Build history of the part. All positions in model axes, mm. A direction names the side the tool comes from. Round coordinates to 2 decimals unless told otherwise and drop trailing zeros. Loops run counter-clockwise (first coordinate to the right, second up) from the corner with the lowest first, then second, coordinate; pieces in that order, holes last. Notation, with made-up numbers: M 84.25,-4.5 L 114.25,-4.5 A26 cw 114.25,18.5 Z; hole C 12.5,65.5 d9. An arc over 180 degrees is marked long. Use one line per item in the form item = value. Start each with the question number.
```python
from build123d import *

# Parameters (mm, degrees)
SKETCH_R        = 1.7
PAD_DEPTH       = 10
SKETCH002_W     = 15
SKETCH002_H     = 10
POCKET_DEPTH    = 7
PAD001_DEPTH    = 3
SKETCH009_R     = 2.8
POCKET003_DEPTH = 2.5
SKETCH010_R     = 1.5
PAD002_DEPTH    = 3
SKETCH011_R     = 1
POCKET004_DEPTH = 24
SKETCH012_R     = 1.8
POCKET005_DEPTH = 11
SKETCH013_R     = 2
POCKET006_DEPTH = 6
FILLET_R        = 2
FILLET001_R     = 2


with BuildPart() as part:
    # Sketch → Pad (new body)
    with BuildSketch(Plane.XY):
        Polygon((-10, 10), (5, 10), (5, 4.942513), (5, -5.057487), (5, -10), (-10, -10), (-10, -5.057487), (-25, -5.057487), (-25, 4.942513), (-10, 4.942513), align=None)
        with Locations((-17.661669, 0)):
            Circle(SKETCH_R, mode=Mode.SUBTRACT)
        with Locations((-7.661669, 0)):
            Circle(SKETCH_R, mode=Mode.SUBTRACT)
    extrude(amount=PAD_DEPTH)

    # Sketch002 (on Face14 of Pad) → Pocket (cut)
    with BuildSketch(Plane.XY.offset(10)):
        with Locations((-17.5, -0.057487)):
            Rectangle(SKETCH002_W, SKETCH002_H)
    extrude(amount=-POCKET_DEPTH, mode=Mode.SUBTRACT)

    # Sketch003 (on Face13 of Pocket) → Pad001 (join)
    with BuildSketch(Plane.XZ.offset(10)):
        with BuildLine():
            ThreePointArc((1.21175, 5.90888), (0, 9.5), (-1.21175, 5.90888))
            Line((-1.21175, 5.90888), (-1.21175, 0))
            Line((-1.21175, 0), (1.21175, 0))
            Line((1.21175, 0), (1.21175, 5.90888))
        make_face()
    extrude(amount=PAD001_DEPTH)

    # Sketch009 (on Face14 of Pad) → Pocket003 (cut)
    with BuildSketch(Plane.XY.offset(10)):
        with Locations((-7.661669, 0)):
            Circle(SKETCH009_R)
    extrude(amount=-POCKET003_DEPTH, mode=Mode.SUBTRACT)

    # Sketch010 (on Face24 of Pocket003) → Pad002 (join)
    with BuildSketch(Plane.XZ.offset(13)):
        with Locations((0, 7.5)):
            Circle(SKETCH010_R)
    extrude(amount=PAD002_DEPTH)

    # Sketch011 (on Face26 of Pad002) → Pocket004 (cut)
    with BuildSketch(Plane.XZ.offset(16)):
        with Locations((0, 7.5)):
            Circle(SKETCH011_R)
    extrude(amount=-POCKET004_DEPTH, mode=Mode.SUBTRACT)

    # Sketch012 (on Face1 of Pocket004) → Pocket005 (cut)
    with BuildSketch(Plane(origin=(-10, 0, 0), x_dir=(0, -1, 0), z_dir=(-1, 0, 0))):
        with Locations((-7.264964, 7)):
            Circle(SKETCH012_R)
    extrude(amount=-POCKET005_DEPTH, mode=Mode.SUBTRACT)

    # Sketch013 (on Face1 of Pocket005) → Pocket006 (cut)
    with BuildSketch(Plane(origin=(-10, 0, 0), x_dir=(0, -1, 0), z_dir=(-1, 0, 0))):
        with Locations((-7.264964, 7)):
            Circle(SKETCH013_R)
    extrude(amount=-POCKET006_DEPTH, mode=Mode.SUBTRACT)

    # Fillet
    fillet_edges = [part.edges().sort_by_distance(p)[0] for p in [
        (5, -10, 5),
    ]]
    fillet(fillet_edges, radius=FILLET_R)

    # Fillet001
    fillet001_edges = [part.edges().sort_by_distance(p)[0] for p in [
        (-25, -0.057487, 3),
    ]]
    fillet(fillet001_edges, radius=FILLET001_R)


solid = part.part
```
Q1. Saw through at B-B (z = 4). Give the cut face in (x, y), and give its area (3 significant figures).
Q2. Wall check: probe 1 along X at (y, z) = (0, 0.9); probe 2 along Y at (x, z) = (-1.75, 7); probe 3 along X at (y, z) = (0, 2). Give the ranges that are in metal, low to high.
Q3. Drop flat-ended pins along their axis: P1, Ø3.5, axis at x = -15.5, z = 1, coming from the -Y side; P2, Ø3.5, axis at y = -12, z = 1.5, coming from the -X side; P3, Ø4.5, axis at x = -7.66, y = 0, coming from the +Z side. Give the stop position or say it passes through.
Q4. Saw through at C-C (x = 0). Give the cut face in (y, z).
Q5. Tool access for faces 4 (the face through (1.212, -11, 3)), 5 (the face through (-15, 0, 3)), 6 (the face through (-18, 4.943, 1)), 7 (the face through (-1.212, -11, 3)): list every direction of +Z, -Z, +X, -X, +Y, -Y with a clear straight run to the whole face (end or side of a thin tool).
Q6. Pull direction Z, two halves, no side cores. Call faces 1 (the face through (1, 7, 7)), 2 (the face through (-6, -1, 7.5)), 3 (the face through (0.07, -11.48, 9.5)): pulls with the +Z half, pulls with the -Z half, needs draft (parallel to the pull), parting line crosses it, or undercut.
Q7. Saw through at D-D (y = -6.75). Give the cut face in (x, z), and give its area (3 significant figures).
Q8. Saw through at A-A (y = 0). Give the cut face in (x, z), and give its area (3 significant figures).
Filled in:
q1.outline = M -10,-10 L -1.21,-10 L -1.21,-13 L 1.21,-13 L 1.21,-10 L 3,-10 A2 ccw 5,-8 L 5,10 L -10,10 Z; hole C -7.66,0 d3.4
q1.area = 297 mm²
q2.probe_1 = -25 to -19.36, -15.96 to -9.36, -5.96 to 5
q2.probe_2 = -13 to 5.46, 9.06 to 10
q2.probe_3 = -24.73 to -19.36, -15.96 to -9.36, -5.96 to 5
q3.P1 = -5.06
q3.P2 = -1.21
q3.P3 = 7.5
q4.outline = M -16,6 L -13,6 L -13,0 L 10,0 L 10,10 L -10,10 L -10,9.5 L -13,9.5 L -13,9 L -16,9 L -16,8.5 L 6.27,8.5 A1.8 cw long 5.54,6.5 L -16,6.5 Z
q5.face_4 = -Z, +X, -Y
q5.face_5 = +Z, -X, +Y, -Y
q5.face_6 = +Z, -Z, -X, +Y
q5.face_7 = -Z, -X, -Y
q6.face_1 = undercut
q6.face_2 = pulls with the +Z half
q6.face_3 = parting line crosses it
q7.outline = M -10,0 L 5,0 L 5,10 L -10,10 Z; hole C 0,7.5 d2
q7.area = 147 mm²
q8.outline = M -25,0 L -19.36,0 L -19.36,3 L -23,3 A2 ccw -25,1 Z; M -15.96,0 L -9.36,0 L -9.36,7.5 L -10,7.5 L -10,3 L -15.96,3 Z; M -5.96,0 L 5,0 L 5,10 L -4.86,10 L -4.86,7.5 L -5.96,7.5 Z; hole C 0,7.5 d2
q8.area = 142 mm²
